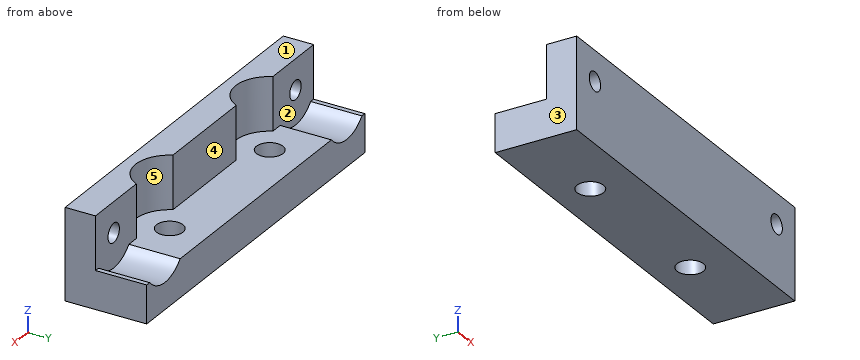
```python
from build123d import *

# Parameters (mm, degrees)
F2_DEPTH      = 5
F3_DEPTH      = 7
F4_D          = 3.5
F4_DEPTH      = 10
F4_TIP        = 1.0515060833
F5_R          = 4.5
F5_R_2        = 1.25
F6_DEPTH      = 6.4
F6_DEPTH_BACK = 2
F7_DEPTH      = 25


with BuildPart() as f2:
    # F1 (on Top) → F2 (new body)
    with BuildSketch(Plane.XY):
        with BuildLine():
            Line((24, 4.75), (-24, 4.75))
            Line((-24, 4.75), (-24, -2))
            Line((-24, -2), (-15.0311288741, -2))
            ThreePointArc((-15.0311288741, -2), (-12.0271124735, 4.3812144397), (-6.5, 0))
            ThreePointArc((-6.5, 0), (-6.6187855603, -1.0271124735), (-6.9688711259, -2))
            Line((-6.9688711259, -2), (6.9688711259, -2))
            ThreePointArc((6.9688711259, -2), (9.9728875265, 4.3812144397), (15.5, 0))
            ThreePointArc((15.5, 0), (15.3812144397, -1.0271124735), (15.0311288741, -2))
            Line((15.0311288741, -2), (24, -2))
            Line((24, -2), (24, 4.75))
        make_face()
        with BuildLine():
            ThreePointArc((-6.5, 0), (-12.0271124735, 4.3812144397), (-15.0311288741, -2))
            Line((-15.0311288741, -2), (-6.9688711259, -2))
            ThreePointArc((-6.9688711259, -2), (-6.6187855603, -1.0271124735), (-6.5, 0))
        make_face()
        with BuildLine():
            Line((-15.0311288741, -2), (-24, -2))
            Line((-24, -2), (-24, -6))
            Line((-24, -6), (24, -6))
            Line((24, -6), (24, -2))
            Line((24, -2), (15.0311288741, -2))
            ThreePointArc((15.0311288741, -2), (11, -4.5), (6.9688711259, -2))
            Line((6.9688711259, -2), (-6.9688711259, -2))
            ThreePointArc((-6.9688711259, -2), (-11, -4.5), (-15.0311288741, -2))
        make_face()
        with BuildLine():
            Line((-6.9688711259, -2), (-15.0311288741, -2))
            ThreePointArc((-15.0311288741, -2), (-11, -4.5), (-6.9688711259, -2))
        make_face()
        with BuildLine():
            ThreePointArc((6.9688711259, -2), (11, -4.5), (15.0311288741, -2))
            Line((15.0311288741, -2), (6.9688711259, -2))
        make_face()
        with BuildLine():
            Line((6.9688711259, -2), (15.0311288741, -2))
            ThreePointArc((15.0311288741, -2), (15.3812144397, -1.0271124735), (15.5, 0))
            ThreePointArc((15.5, 0), (9.9728875265, 4.3812144397), (6.9688711259, -2))
        make_face()
    extrude(amount=-F2_DEPTH)

    # F1 (on Top) → F3 (join)
    with BuildSketch(Plane.XY):
        with BuildLine():
            Line((-15.0311288741, -2), (-24, -2))
            Line((-24, -2), (-24, -6))
            Line((-24, -6), (24, -6))
            Line((24, -6), (24, -2))
            Line((24, -2), (15.0311288741, -2))
            ThreePointArc((15.0311288741, -2), (11, -4.5), (6.9688711259, -2))
            Line((6.9688711259, -2), (-6.9688711259, -2))
            ThreePointArc((-6.9688711259, -2), (-11, -4.5), (-15.0311288741, -2))
        make_face()
    extrude(amount=F3_DEPTH)

    # F4
    with Locations(Plane.XY):
        with Locations((-11, 0), (11, 0)):
            Hole(F4_D / 2, depth=F4_DEPTH)
            with Locations((0, 0, -(F4_DEPTH + F4_TIP / 2))):  # 118° drill point
                Cone(0, F4_D / 2, F4_TIP, mode=Mode.SUBTRACT)

    # F5 (on Front) → F6 (cut, two sides)
    with BuildSketch(Plane.XZ) as f6_sk:
        with Locations((20, 3)):
            Circle(F5_R)
        with Locations((20, 3)):
            Circle(F5_R_2, mode=Mode.SUBTRACT)
        with Locations((-20, 3)):
            Circle(F5_R)
        with Locations((-20, 3)):
            Circle(F5_R_2, mode=Mode.SUBTRACT)
    extrude(amount=-F6_DEPTH, mode=Mode.SUBTRACT)
    extrude(f6_sk.sketch, amount=F6_DEPTH_BACK, mode=Mode.SUBTRACT)

    # F5 (on Front) → F7 (cut)
    with BuildSketch(Plane.XZ):
        with Locations((-20, 3)):
            Circle(F5_R_2)
        with Locations((20, 3)):
            Circle(F5_R_2)
    extrude(amount=F7_DEPTH, mode=Mode.SUBTRACT)


solid = f2.part
```
Design review of the part built by this model. Coordinates are the model's own, in mm. Face numbers are marked on the shaded views. A direction names the side the tool comes from. Give positions to 0.01 mm unless a question says otherwise; leave off trailing zeros. Loops run counter-clockwise (first coordinate to the right, second up) from the corner with the lowest first, then second, coordinate; pieces in that order, holes last. Notation, with made-up numbers: (3, 20.25) -> (30, 20.25) arc R22 cw to (30, 26.25) -> close; hole circle Ø3 at (59.5, 73). An arc over 180 degrees is marked (long way). Write each question's results on one line, items separated by ' | '.
Q1. Take a section at A-A, the plane x = -20. Write out the cut boundary in (y, z).
Reply:
outline: (-6, -5) -> (4.75, -5) -> (4.75, -1.5) -> (-2, -1.5) -> (-2, 1.75) -> (-6, 1.75) -> close; (-6, 4.25) -> (-2, 4.25) -> (-2, 7) -> (-6, 7) -> close
Q2. Wall thickness on L1, parallel to X at y = -4.9, z = 3; L2, parallel to Y at x = 11, z = -3; L3, parallel to X at y = -3.25, z = 3: over which ranges is each line inside the solid? List them lowest first.
Reply:
L1: x = -24 to -21.25, -18.75 to 18.75, 21.25 to 24 | L2: y = -6 to -1.75, 1.75 to 4.75 | L3: x = -24 to -21.25, -18.75 to -14.11, -7.89 to 7.89, 14.11 to 18.75, 21.25 to 24
Q3. Machinability: for the marked faces 1 and 2, which of the approach directions +Z, -Z, +X, -X, +Y, -Y give a long, thin tool a straight path to every point of the face, cutting with its end or side? Answer none if there is none.
Reply:
face 1: +Z, +X, -X, +Y, -Y | face 2: +Z, +Y
Q4. The part is to be moulded in two halves that separate along X. For the marked faces 3, 4 and 5, say which applies: +X half, -X half, draft (parallel to the pull), parting line (faces both ways), or undercut.
Reply:
face 3: -X half | face 4: draft | face 5: undercut
Q5. Take a section at C-C, the plane y = -0.5. Write out the cut boundary in (x, z), plus the area to 3 significant figures.
Reply:
outline: (-24, -5) -> (-12.68, -5) -> (-12.68, 0) -> (-16.65, 0) arc R4.5 cw to (-23.35, 0) -> (-24, 0) -> close; (-9.32, -5) -> (9.32, -5) -> (9.32, 0) -> (-9.32, 0) -> close; (12.68, -5) -> (24, -5) -> (24, 0) -> (23.35, 0) arc R4.5 cw to (16.65, 0) -> (12.68, 0) -> close | area: 193 mm²
Q6. Take a section at B-B, the plane z = -3.5. Write out the cut boundary in (x, y), plus the area to 3 significant figures.
Reply:
outline: (-24, -6) -> (24, -6) -> (24, 4.75) -> (-24, 4.75) -> close; hole circle Ø3.5 at (-11, 0); hole circle Ø3.5 at (11, 0) | area: 497 mm²
Q7. Take a section at D-D, the plane x = 3.5. Write out the cut boundary in (y, z).
Reply:
outline: (-6, -5) -> (4.75, -5) -> (4.75, 0) -> (-2, 0) -> (-2, 7) -> (-6, 7) -> close
Q8. For pin 1 Ø0.7 at (x, y) = (-24, 2) entering from +Z; pin 2 Ø5 at (x, z) = (-6, 4) entering from +Y, all flat-tipped, find the tip position at first contact; note any pin that passes through.
Reply:
pin 1: stops at z = 0 | pin 2: stops at y = -2
